For this review, use the dimensioned drawing (mm, ordinates from the lowest corner) and the shaded views. Give positions to 0.01 mm unless a question says otherwise; leave off trailing zeros. Loops run counter-clockwise (first coordinate to the right, second up) from the corner with the lowest first, then second, coordinate; pieces in that order, holes last. Notation, with made-up numbers: (3, 36) -> (44, 36) arc R21 cw to (44, 66) -> close; hole circle Ø6 at (77.25, 31). An arc over 180 degrees is marked (long way). Write each question's results on one line, items separated by ' | '. Start each with the question number.
Q1. We need section A-A (x = 70.25). Write out the cut boundary in (y, z).
Q2. We need section B-B (z = 28). Write out the cut boundary in (x, y).
Q3. We need section C-C (x = 45.5). Write out the cut boundary in (y, z), plus the area to 3 significant figures.
Q4. Wall thickness on L1, parallel to Z at x = 70.25, y = 2; L2, parallel to X at y = 8.05, z = 28; L3, parallel to Z at x = 45.5, y = 9.1: over which ranges is each line inside the solid? List them lowest first. Write a range as [from, to].
Q5. Insertion check: pin 1 Ø6.5 at (x, z) = (45.5, 28) entering from -Y; pin 2 Ø3 at (x, z) = (70.25, 42.29) entering from +Y. Each pin has a flat end and moves straight along its axis. Give the tip position at first contact, or say it passes through.
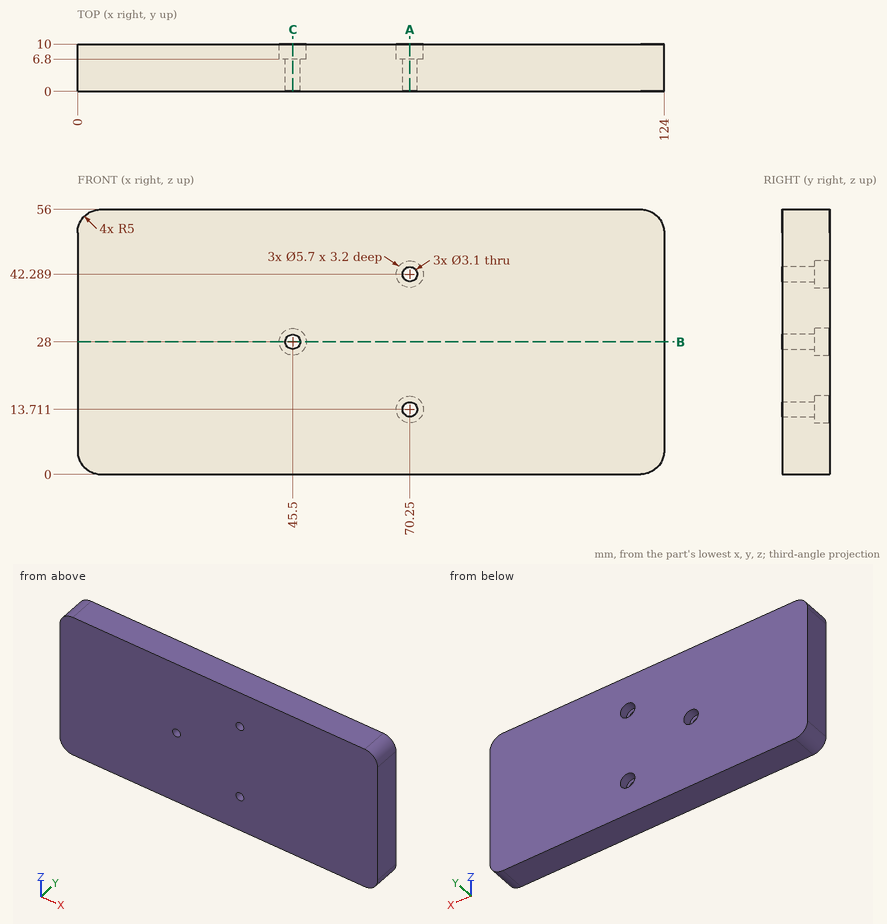
Output:
1) outline: (0, 0) -> (10, 0) -> (10, 10.86) -> (6.8, 10.86) -> (6.8, 12.16) -> (0, 12.16) -> close; (0, 15.26) -> (6.8, 15.26) -> (6.8, 16.56) -> (10, 16.56) -> (10, 39.44) -> (6.8, 39.44) -> (6.8, 40.74) -> (0, 40.74) -> close; (0, 43.84) -> (6.8, 43.84) -> (6.8, 45.14) -> (10, 45.14) -> (10, 56) -> (0, 56) -> close
2) outline: (0, 0) -> (43.95, 0) -> (43.95, 6.8) -> (42.65, 6.8) -> (42.65, 10) -> (0, 10) -> close; (47.05, 0) -> (124, 0) -> (124, 10) -> (48.35, 10) -> (48.35, 6.8) -> (47.05, 6.8) -> close
3) outline: (0, 0) -> (10, 0) -> (10, 25.15) -> (6.8, 25.15) -> (6.8, 26.45) -> (0, 26.45) -> close; (0, 29.55) -> (6.8, 29.55) -> (6.8, 30.85) -> (10, 30.85) -> (10, 56) -> (0, 56) -> close | area: 521 mm2
4) L1: [0, 12.16], [15.26, 40.74], [43.84, 56] | L2: [0, 42.65], [48.35, 124] | L3: [0, 25.15], [30.85, 56]
5) pin 1: y = 0 | pin 2: through
